Geometry check sheet. Reference: the model listing, model coordinates, mm. A direction names the side the tool comes from. Give positions to 0.01 mm unless a question says otherwise; leave off trailing zeros. Loops run counter-clockwise (first coordinate to the right, second up) from the corner with the lowest first, then second, coordinate; pieces in that order, holes last. Notation, with made-up numbers: (63.5, -23.5) -> (100.5, -23.5) arc R12 cw to (100.5, -3.5) -> close; hole circle Ø4 at (28.5, 74.5). An arc over 180 degrees is marked (long way). Write item = value, one per line.
```python
from build123d import *

# Parameters (mm, degrees)
SKETCH_1_R      = 1.5
EXTRUDE_1_DEPTH = 3


with BuildPart() as part:
    # 草图1 → 凸台-拉伸1 (new body)
    with BuildSketch(Plane(origin=(0, 0, 0), x_dir=(1, 0, 0), z_dir=(0, 1, 0))):
        Polygon((38, -9), (38, 9), (7, 9), (-8, 27), (-24, 27), (-37, 2), (-37, -2), (-24, -27), (-8, -27), (7, -9), align=None)
        with Locations(Location((-21, 20, 0), (0, 0, 270))):
            Circle(SKETCH_1_R, mode=Mode.SUBTRACT)
        with Locations(Location((-11, 20, 0), (0, 0, 270))):
            Circle(SKETCH_1_R, mode=Mode.SUBTRACT)
        with Locations(Location((-11, -20, 0), (0, 0, 90))):
            Circle(SKETCH_1_R, mode=Mode.SUBTRACT)
        with Locations(Location((-21, -20, 0), (0, 0, 90))):
            Circle(SKETCH_1_R, mode=Mode.SUBTRACT)
        with Locations(Location((-32, 0, 0), (0, 0, 270))):
            Circle(SKETCH_1_R, mode=Mode.SUBTRACT)
        with BuildLine():
            Line((6.92820323, 4), (27.25, 4))
            Line((27.25, 4), (27.25, -4))
            Line((27.25, -4), (6.92820323, -4))
            ThreePointArc((6.92820323, -4), (-8, 0), (6.92820323, 4))
        make_face(mode=Mode.SUBTRACT)
    extrude(amount=EXTRUDE_1_DEPTH)


solid = part.part
```
Item 1: Thickness scan on L1, parallel to X at y = 1, z = 0; L2, parallel to X at y = 1, z = 20; L3, parallel to Z at x = 13, y = 0.55. Record the ranges inside material, lowest first. Write a range as [from, to].
Answer:
L1 = [-37, -33.5], [-30.5, -8], [27.25, 38]
L2 = [-27.64, -22.5], [-19.5, -12.5], [-9.5, -2.17]
L3 = [-9, -4], [4, 9]
Item 2: Section check B-B, the plane z = -20. Record the cut outline in (x, y), plus the area to 3 significant figures.
Answer:
outline = (-27.64, 0) -> (-22.5, 0) -> (-22.5, 3) -> (-27.64, 3) -> close; (-19.5, 0) -> (-12.5, 0) -> (-12.5, 3) -> (-19.5, 3) -> close; (-9.5, 0) -> (-2.17, 0) -> (-2.17, 3) -> (-9.5, 3) -> close
area = 58.4 mm^2
Item 3: Section check D-D, the plane y = 1.05. Record the cut outline in (x, z), plus the area to 3 significant figures.
Answer:
outline = (-37, -2) -> (-24, -27) -> (-8, -27) -> (7, -9) -> (38, -9) -> (38, 9) -> (7, 9) -> (-8, 27) -> (-24, 27) -> (-37, 2) -> close; hole circle Ø3 at (-32, 0); hole circle Ø3 at (-21, -20); hole circle Ø3 at (-21, 20); hole circle Ø3 at (-11, -20); hole circle Ø3 at (-11, 20); hole (6.93, -4) -> (27.25, -4) -> (27.25, 4) -> (6.93, 4) arc R8 ccw (long way) to start
area = 1,950 mm^2
Item 4: Section check C-C, the plane x = -11. Record the cut outline in (y, z), plus the area to 3 significant figures.
Answer:
outline = (0, -27) -> (3, -27) -> (3, -21.5) -> (0, -21.5) -> close; (0, -18.5) -> (3, -18.5) -> (3, 18.5) -> (0, 18.5) -> close; (0, 21.5) -> (3, 21.5) -> (3, 27) -> (0, 27) -> close
area = 144 mm^2
Item 5: Draft check along X on faces 1 (the cylindrical face through (-22.01, 1.48, 21.11)), 2 (the flat face through (-0.395, 1.479, -17.874)), 3 (the flat face through (27.25, 1, 0)), 4 (the flat face through (23, 1, -9)). Enter one of: +X half, -X half, draft (parallel to the pull), parting line (faces both ways), or undercut.
Answer:
face_1 = undercut
face_2 = +X half
face_3 = undercut
face_4 = draft
Item 6: Gauge pin test, flat ends, axial feed: pin 1 (5 mm diameter, centred on x = -11, z = -20, fed in from -Y); pin 2 (1 mm diameter, centred on x = 23.5, y = 2, fed in from +Z); pin 3 (2.5 mm diameter, centred on x = -32, z = 0, fed in from -Y) (3 decimals); pin 4 (1.5 mm diameter, centred on x = 23, y = 1.5, fed in from -Z). Record the tip position at first contact, or that the pin passes through.
Answer:
pin_1 = 0
pin_2 = 9
pin_3 = through
pin_4 = -9
Item 7: Section check A-A, the plane x = 0. Record the cut outline in (y, z).
Answer:
outline = (0, -17.4) -> (3, -17.4) -> (3, -8) -> (0, -8) -> close; (0, 8) -> (3, 8) -> (3, 17.4) -> (0, 17.4) -> close
Item 8: Tool access check on faces 5 (the flat face through (-16, 1, 27)), 6 (the flat face through (22, 1, 9)), 7 (the flat face through (17, 1, 4)). Record the directions out of +Z, -Z, +X, -X, +Y, -Y that give a thin tool (end or side, any length) a straight path to the whole face; none if there is none.
Answer:
face_5 = +Z, +X, -X, +Y, -Y
face_6 = +Z, +X, +Y, -Y
face_7 = +Y, -Y
